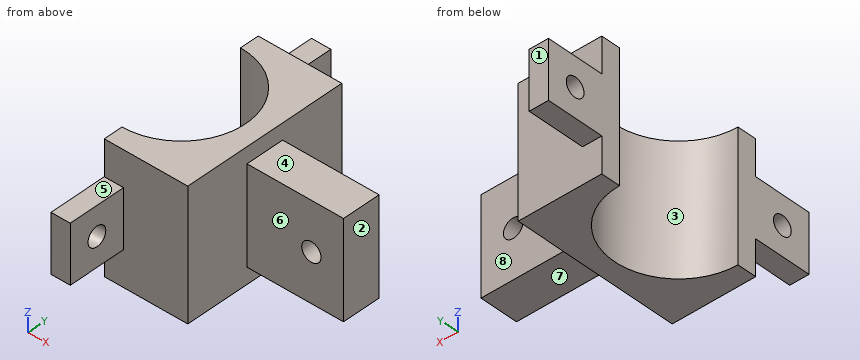
from build123d import *

# Parameters (mm, degrees)
EXTRUDE_1_DEPTH     = 20
SKETCH_7_W          = 9
SKETCH_7_H          = 12
SKETCH_7_R          = 1.5
EXTRUDE_3_DEPTH     = 3
EXTRUDE_4_DEPTH     = 15
SKETCH_9_R          = 1.5
CUT_EXTRUDE_1_DEPTH = 15
SKETCH_6_R          = 1.5
EXTRUDE_2_DEPTH     = 3


with BuildPart() as part:
    # Эскиз1 → Бобышка-Вытянуть1 (new body)
    with BuildSketch(Plane.XY):
        with BuildLine():
            Line((0, 10), (0, 13))
            Line((0, 13), (13, 13))
            Line((13, 13), (13, -13))
            Line((13, -13), (0, -13))
            Line((0, -13), (0, -10))
            ThreePointArc((0, -10), (10, 0), (0, 10))
        make_face()
    extrude(amount=EXTRUDE_1_DEPTH)

    # Эскиз7 → Бобышка-Вытянуть3 (add)
    # profile 1 of 2: a face of its own
    with BuildSketch(Plane.ZY):
        with Locations((10, 16)):
            Rectangle(SKETCH_7_W, SKETCH_7_H)
        with Locations((10, 17.5)):
            Circle(SKETCH_7_R, mode=Mode.SUBTRACT)
    # profile 2 of 2: a face of its own
    with BuildSketch(Plane.ZY):
        with Locations((10, -16)):
            Rectangle(SKETCH_7_W, SKETCH_7_H)
        with Locations((10, -17.5)):
            Circle(SKETCH_7_R, mode=Mode.SUBTRACT)
    extrude(amount=-EXTRUDE_3_DEPTH)

    # Эскиз8 → Бобышка-Вытянуть4 (add)
    with BuildSketch(Plane(origin=(13, 0, 0), x_dir=(0, 0, -1), z_dir=(1, 0, 0))):
        Polygon((-17.5, 3), (-17.5, -3), (-2.5, -3), (-2.5, 3), (-10, 3), align=None)
    extrude(amount=EXTRUDE_4_DEPTH)

    # Эскиз9 → Вырез-Вытянуть1 (cut)
    with BuildSketch(Plane(origin=(0, 3, 0), x_dir=(1, 0, 0), z_dir=(0, 1, 0))):
        with Locations(Location((23, -10, 0), (0, 0, 270))):
            Circle(SKETCH_9_R)
    extrude(amount=-CUT_EXTRUDE_1_DEPTH, mode=Mode.SUBTRACT)

    # Эскиз6 → Бобышка-Вытянуть2 (add)
    # profile 1 of 2: a face of its own
    with BuildSketch(Plane.ZY):
        Polygon((10, 10), (5.5, 10), (5.5, 22), (14.5, 22), (14.5, 10), align=None)
        with Locations((10, 17.5)):
            Circle(SKETCH_6_R, mode=Mode.SUBTRACT)
    # profile 2 of 2: a face of its own
    with BuildSketch(Plane.ZY):
        Polygon((10, -10), (5.5, -10), (5.5, -22), (14.5, -22), (14.5, -10), align=None)
        with Locations((10, -17.5)):
            Circle(SKETCH_6_R, mode=Mode.SUBTRACT)
    extrude(amount=-EXTRUDE_2_DEPTH)


solid = part.part
Geometry: final body of the model. Coordinates: model frame, mm. Face numbers are marked on the shaded views. A direction names the side the tool comes from. Give positions to 0.01 mm unless a question says otherwise; leave off trailing zeros. Write each loop counter-clockwise with the first axis right and the second up, starting at its lowest first coordinate (ties: lowest second). Pieces come first, ordered by that corner, then holes. Notation, with made-up numbers: M 14,66.5 L 34,66.5 A17 ccw 34,88.5 Z; hole C -9,-25.5 d8. An arc over 180 degrees is marked long. Answer in a Markdown table with one row per item. Add a question column.
(1) Section C-C on x = 23. Return loops of the section in (y, z).
(2) Section B-B on y = 17.5. Return loops of the section in (x, z), and give its area (3 significant figures).
(3) Reachability of the marked faces 4, 5, 6, 7 and 8 from +Z, -Z, +X, -X, +Y, -Y: full face, straight path, thin tool, end or side. Return the list, or none.
(4) Section D-D on z = 7. Return loops of the section in (x, y).
(5) First-contact query: pin 1 (1.5 mm diameter, centred on x = 4.5, z = 15.5, fed in from +Y); pin 2 (3 mm diameter, centred on y = 16.5, z = 9, fed in from +X); pin 3 (2.5 mm diameter, centred on x = 1, y = 17.5, fed in from +Z). Flat tips, straight axial feed; report the tip coordinate or a pass-through.
(6) Section A-A on z = 10. Return loops of the section in (x, y).
(7) Ray query, line 1 (Y direction, x = 0.7, z = 10); line 2 (Y direction, x = 1.5, z = 10); line 3 (Y direction, x = 17.25, z = 3.25). Return the intervals inside material, ascending.
(8) Mould query, pull axis Y, two halves, no side actions, for the marked faces 1, 2 and 3. Classes: +Y half, -Y half, draft (parallel to the pull), parting line (faces both ways), or undercut.
Result set:
| question | item | result |
|---|---|---|
| 1 | outline | M -3,2.5 L 3,2.5 L 3,8.5 L -3,8.5 Z; M -3,11.5 L 3,11.5 L 3,17.5 L -3,17.5 Z |
| 2 | outline | M 0,5.5 L 3,5.5 L 3,8.5 L 0,8.5 Z; M 0,11.5 L 3,11.5 L 3,14.5 L 0,14.5 Z |
| 2 | area | 18.0 mm^2 |
| 3 | face 4 | +Z, +X, +Y, -Y |
| 3 | face 5 | +Z, +X, -X, -Y |
| 3 | face 6 | +Z, -Z, +X, -Y |
| 3 | face 7 | -Z, +X, +Y, -Y |
| 3 | face 8 | +Z, -Z, +X, +Y |
| 4 | outline | M 0,-22 L 3,-22 L 3,-13 L 13,-13 L 13,-3 L 28,-3 L 28,3 L 13,3 L 13,13 L 3,13 L 3,22 L 0,22 L 0,10 A10 cw 0,-10 Z |
| 5 | pin 1 | stops at y = 13 |
| 5 | pin 2 | stops at x = 3 |
| 5 | pin 3 | stops at z = 14.5 |
| 6 | outline | M 0,-22 L 3,-22 L 3,-19 L 0,-19 Z; M 0,-16 L 3,-16 L 3,-13 L 13,-13 L 13,-3 L 21.5,-3 L 21.5,3 L 13,3 L 13,13 L 3,13 L 3,16 L 0,16 L 0,10 A10 cw 0,-10 Z; M 0,19 L 3,19 L 3,22 L 0,22 Z; M 24.5,-3 L 28,-3 L 28,3 L 24.5,3 Z |
| 7 | line 1 | y = -22 to -19, -16 to -9.98, 9.98 to 16, 19 to 22 |
| 7 | line 2 | y = -22 to -19, -16 to -9.89, 9.89 to 16, 19 to 22 |
| 7 | line 3 | y = -3 to 3 |
| 8 | face 1 | +Y half |
| 8 | face 2 | draft |
| 8 | face 3 | undercut |
